Model file for the job. Use its own axes, mm. A direction names the side the tool comes from. Give positions to 0.01 mm unless a question says otherwise; leave off trailing zeros. Order: outer loops, then holes, each group sorted by start corner. A loop starts at its lowest first (then second) coordinate and runs counter-clockwise, first axis right, second up. Notation, with made-up numbers: (55, 76.5) - (94, 76.5) arc R14 ccw to (94, 86.5) - close; hole circle Ø8 at (-30, 55.25). An arc over 180 degrees is marked (long way). Use CSV: the item, a comma, the result in double quotes. Start each with the question number.
(1) Probe L1, parallel to X at y = -1.05, z = -1.85; L2, parallel to Y at x = -1.25, z = 1.05; L3, parallel to Y at x = 1.5, z = -0.25. List the from-to ranges inside material, lowest first.
(2) Pull direction Y, two halves, no side cores. Call faces 1 (the flat face through (-2, -1, 1)), 2 (the flat face through (-1.22, -0.49, 0.87)), 3 (the cylindrical face through (-0.862, -0.596, 2.685)): +Y half, -Y half, draft (parallel to the pull), parting line (faces both ways), or undercut.
(3) Drop flat-ended pins along their axis: pin 1 Ø3 at (x, y) = (2, 1) entering from -Z; pin 2 Ø1 at (y, z) = (-1.5, -1.5) entering from +X. Give the stop position or say it passes through.
(4) Band-saw the part on A-A, the plane x = 8.5. Give the cut face in (y, z), then the cut area to 3 significant figures.
(5) Tool access for faces 4 (the flat face through (16, 0, 0)), 5 (the flat face through (-1, 1, 0)), 6 (the flat face through (0, 2, 0)): list every direction of +Z, -Z, +X, -X, +Y, -Y with a clear straight run to the whole face (end or side of a thin tool).
Autodesk Inventor part; units mm, degrees
ref_plane "Work Plane1" through (29, 0, 0) normal (0, -1, 0) x (1, 0, 0)
ref_plane "YZ Plane" through (0, 0, 0) normal (1, 0, 0) x (0, 1, 0)
ref_plane "XZ Plane" through (0, 0, 0) normal (0, 1, 0) x (-1, 0, 0)
sketch "Skizze1" plane through (0, 0, 0) normal (0, 0, 1) x (1, 0, 0)
  line L0 (0.1667, 0) -> (16, 0)
  line L1 (16, 0) -> (16, 1.5)
  line L2 (16, 1.5) -> (1.5, 1.5)
  line L3 (1.5, 1.5) -> (1.1932, 1.5)
  line L4 (1.1932, 1.5) -> (0, 1.5)
  line L5 (0, 1.5) -> (0, 2.75)
  line L6 (0, 2.75) -> (-2, 2.75)
  line L7 (-2, 2.75) -> (-2, 1.1547)
  line L8 (-2, 1.1547) -> (-0.5, 1.1547)
  line L9 (-0.5, 1.1547) -> (0.1667, 0)
  line L10 (-5.6, 0) -> (19.6, 0)
  line L11 (0, -0.55) -> (0, 3.3)
  line L12 (1.5, 1.5) -> (0, 1.5) construction
  dimension "d1" = 14.5
  dimension "d2" = 0.3068
  dimension "d3" = 2
  dimension "d4" = 1.5
  dimension "d5" = 60
  dimension "d6" = 3
  dimension "d7" = 3
  dimension "d8" = 2.3094
  dimension "d9" = 5.5
  dimension "d26" = 16
revolve "Körper" add sketch "Skizze1" angle 360 about axis through (0.1667, 0, 0) along (1, 0, 0) contours L9 L11 L4 L3 L2 L1 L0 | L9 L8 L7 L6 L5 L11
sketch "Skizze2" plane through (-2, 0, 0) normal (-1, 0, 0) x (0, 0, 1)
  circle A0 centre (0, 0) radius 1.1547
  line L0 (0, -3.85) -> (0, 3.85)
  line L1 (-3.85, 0) -> (3.85, 0)
  line L2 (1.1547, 0) -> (0.5774, -1)
  line L3 (0.5774, -1) -> (-0.5774, -1)
  line L4 (-0.5774, -1) -> (-1.1547, 0)
  line L5 (-1.1547, 0) -> (-0.5774, 1)
  line L6 (-0.5774, 1) -> (0.5774, 1)
  line L7 (0.5774, 1) -> (1.1547, 0)
  point P0 (0, 0)
extrude "Loch" add sketch "Skizze2" against normal up to next contours L7 A0 | A0 L2 | L6 L0 A0 | A0 L0 L3 | L0 L6 A0 | A0 L3 L0 | L4 A0 | A0 L5
fillet "Rundung1" radius 0.3 1 edges at (-2, -2.75, 0)
thread "Gewinde"
chamfer "Fase1" distance 0.3067 distance2 0.3067 1 edges at (16, -1.5, 0) measured on face at (16, -0.4645, -0.4115)
ref_plane "Work Plane1" through (29, 0, 0) normal (0, -1, 0) x (1, 0, 0)
fillet "Fillet2" radius 0.1 1 edges at (0, -1.5, 0)
equation "\"d1\" = GEL"
equation "\"d3\" = KOH"
equation "\"d4\" = INTI"
equation "\"d6\" = GD"
equation "\"d7\" = BDM"
equation "\"d8\" = 1.1547 * SW"
equation "\"d9\" = KOD"
equation "\"d26\" = NLG"
equation "\"d30\" = R"
equation "\"d17\" = RR"
equation "\"d13\" = GEL"
equation "\"d15\" = -0.5 * SPD + 0.5 * GD"
equation "\"d16\" = GUL"
equation "\"GD\" = NND"
equation "\"NLG\" = 16"
equation "\"GEL\" = 14.5"
equation "\"KOD\" = 5.5"
equation "\"KOH\" = 2"
equation "\"INTI\" = 1.5"
equation "\"GAL\" = 0.61345 * PTC"
equation "\"GUL\" = 0.61345 * PTC"
equation "\"BDM\" = NND"
equation "\"SW\" = 2"
equation "\"RR\" = 0.3"
equation "\"SPD\" = NND - 1.2269 * PTC"
equation "\"R\" = 0.1"
equation "\"TOA\" = 30deg"
equation "\"GD1\" = THREADDIA - 1.2269 * PTC"
equation "\"THREADDIA\" = 3"
equation "\"FAWI\" = 45deg"
equation "\"ANG\" = 120deg"
equation "\"PTC\" = 0.5"
equation "\"NND\" = 3"
equation "\"E0\" = 1.155 * SW"
properties part number "DIN 7984 - M3 x 16" material "Stahl, weich"
Answer block:
1,L1,"x = -2 to 0"
1,L2,"y = -2.54 to -0.18, 0.18 to 2.54"
1,L3,"y = -1.48 to 1.48"
2,face 1,"draft"
2,face 2,"undercut"
2,face 3,"parting line"
3,pin 1,"stops at z = -1.5"
3,pin 2,"stops at x = 0"
4,outline,"circle Ø3 at (0, 0)"
4,area,"7.07 mm2"
5,face 4,"+Z, -Z, +X, +Y, -Y"
5,face 5,"-X"
5,face 6,"+X"
